```python
from build123d import *

# Parameters (mm, degrees)
F4_R      = 25.019
F4_R_2    = 18.669
F11_DEPTH = 12.7
F12_DEPTH = 63.5
F13_R     = 3.175
F13_R_2   = 18.669
F14_DEPTH = 7.62


with BuildPart() as f10:
    # F10: sweep along a path in F9
    with BuildLine(Plane(origin=(0, 0, 0), x_dir=(0.8667959165, 0, 0.4986630517), z_dir=(-0.4986630517, 0, 0.8667959165))) as f10_path:
        ThreePointArc((0, 0), (2.3065003197, 12.6070261986), (3.0790769281, 25.4))
    # F4 (on 3pt) → F10 (sweep)
    with BuildSketch(Plane(origin=(0, 0, 0), x_dir=(0.9804839079, -0.1848249753, -0.0670151833), z_dir=(-0.1965993547, -0.9217625069, -0.3342193511))):
        Circle(F4_R)
        Circle(F4_R_2, mode=Mode.SUBTRACT)
    sweep(path=f10_path.line)

    # F11 (add): a face of the model
    f11_faces = [f10.faces().sort_by_distance(p)[0] for p in [
        (-23.8368931593, 4.4933457387, 1.6292299652),
    ]]
    extrude(f11_faces, amount=F11_DEPTH)

    # F12 (add): a face of the model
    f12_faces = [f10.faces().sort_by_distance(p)[0] for p in [
        (-21.6002276868, 25.0204927062, 2.9159716408),
    ]]
    extrude(f12_faces, amount=F12_DEPTH)

    # F13 (on face) → F14 (join)
    with BuildSketch(Plane(origin=(-0.2452994322, 86.4481864715, 19.4520382221), x_dir=(-0.9999961682, -0.0027007768, -0.0006077121), z_dir=(-0.0027683044, 0.9756031265, 0.2195242038))):
        with BuildLine():
            Line((-28.1384539053, -35.8279679991), (22.6615460947, -35.8279679991))
            ThreePointArc((22.6615460947, -35.8279679991), (27.1516741552, -33.9680960597), (29.0115460947, -29.4779679991))
            Line((29.0115460947, -29.4779679991), (29.0115460947, 21.3220320009))
            ThreePointArc((29.0115460947, 21.3220320009), (27.1516741552, 25.8121600614), (22.6615460947, 27.6720320009))
            Line((22.6615460947, 27.6720320009), (-28.1384539053, 27.6720320009))
            ThreePointArc((-28.1384539053, 27.6720320009), (-32.6285819658, 25.8121600614), (-34.4884539053, 21.3220320009))
            Line((-34.4884539053, 21.3220320009), (-34.4884539053, -29.4779679991))
            ThreePointArc((-34.4884539053, -29.4779679991), (-32.6285819658, -33.9680960597), (-28.1384539053, -35.8279679991))
        make_face()
        with Locations((-28.1384539053, -29.4779679991)):
            Circle(F13_R, mode=Mode.SUBTRACT)
        with Locations((22.6615460947, -29.4779679991)):
            Circle(F13_R, mode=Mode.SUBTRACT)
        with Locations((-28.1384539053, 21.3220320009)):
            Circle(F13_R, mode=Mode.SUBTRACT)
        with Locations((-2.7384539053, -4.0779679991)):
            Circle(F13_R_2, mode=Mode.SUBTRACT)
        with Locations((22.6615460947, 21.3220320009)):
            Circle(F13_R, mode=Mode.SUBTRACT)
    extrude(amount=-F14_DEPTH)


solid = f10.part
```
Build history of the part. All positions in model axes, mm. Give positions to 0.01 mm unless a question says otherwise; leave off trailing zeros. Return JSON: item names as keys, results as strings.
Q1. Wall check: probe 1 along X at (y, z) = (3, 15.5); probe 2 along X at (y, z) = (54, 4); probe 3 along Z at (x, y) = (-8, 25). Give the ranges that are in metal, low to high. Write a range as from..to.
Answer list:
{"probe 1": "x = -19.08..-9.74, 11.57..20.85", "probe 2": "x = -22.13..-15.67, 20.85..27.31", "probe 3": "z = -20.42..-13.35, 17.15..24.65"}
Q2. Flat gauge pins, fed straight in: pin 1 (4 mm diameter, centred on y = 28, z = 20.5, fed in from +X); pin 2 (6 mm diameter, centred on y = 64, z = 34.5, fed in from -X); pin 3 (3 mm diameter, centred on x = -11, y = 79.5, fed in from -Z). Where does each tip first touch, or does it go through?
Answer list:
{"pin 1": "stops at x = 21.94", "pin 2": "stops at x = -11.53", "pin 3": "stops at z = -8.84"}
Q3. Two-plate mould, pull along Z, no slides. Class faces 1 (the face through (32.34, 77.19, 43.88)), 2 (the face through (16.228, -7.151, -8.558)), 3 (the face through (2.859, 90.657, -16.325)), 4 (the face through (28.59, 90.01, -13.14)): pulls with the +Z half, pulls with the -Z half, needs draft (parallel to the pull), parting line crosses it, or undercut.
Answer list:
{"face 1": "pulls with the +Z half", "face 2": "undercut", "face 3": "pulls with the -Z half", "face 4": "undercut"}
Q4. Band-saw the part on A-A (y = 77). Count the separate pieces of the cut face and the enclosed holes in it, then the cut area to 3 significant figures.
Answer list:
{"separate pieces": "1", "enclosed holes": "3", "area": "1,650 mm^2"}
